```python
from build123d import *

# Parameters (mm, degrees)
SKETCH1_W           = 55.5
SKETCH1_H           = 25
BOSS_EXTRUDE1_DEPTH = 70
SKETCH2_W           = 43.5
SKETCH2_H           = 150
CUT_EXTRUDE1_DEPTH  = 20
SKETCH3_R           = 2
CUT_EXTRUDE2_DEPTH  = 78.910605825
FILLET1_R           = 3
CHAMFER1_SIZE       = 6


with BuildPart() as part:
    # Sketch1 → Boss-Extrude1 (new, symmetric)
    with BuildSketch(Plane.XY):
        Rectangle(SKETCH1_W, SKETCH1_H)
    extrude(amount=BOSS_EXTRUDE1_DEPTH, both=True)

    # Sketch2 → Cut-Extrude1 (cut)
    with BuildSketch(Plane(origin=(0, 12.5, 0), x_dir=(1, 0, 0), z_dir=(0, 1, 0))):
        Rectangle(SKETCH2_W, SKETCH2_H)
    extrude(amount=-CUT_EXTRUDE1_DEPTH, mode=Mode.SUBTRACT)

    # Sketch3 → Cut-Extrude2 (cut, through all)
    with BuildSketch(Plane(origin=(0, -7.5, 0), x_dir=(1, 0, 0), z_dir=(0, 1, 0))):
        with Locations(Location((0, 0, 0), (0, 0, 270))):
            Circle(SKETCH3_R)
    extrude(amount=-CUT_EXTRUDE2_DEPTH, mode=Mode.SUBTRACT)

    # Fillet1
    fillet1_edges = [part.edges().sort_by_distance(p)[0] for p in [
        (27.75, -12.5, 0),
        (-27.75, -12.5, 0),
    ]]
    fillet(fillet1_edges, radius=FILLET1_R)

    # Chamfer1
    # the kernel refuses this chamfer: 6 mm, written as the material it takes off along each edge
    with BuildSketch(Plane(origin=(-6.319902072, 12.5, -70), x_dir=(0, -0.9996219169112968, -0.027495876610586778), z_dir=(-1, 0, 0)), Plane(origin=(43.180097928, 12.5, -70), x_dir=(0, -0.9996219169112968, -0.027495876610586778), z_dir=(-1, 0, 0))) as chamfer1_piece_1:
        Polygon((CHAMFER1_SIZE * 0.999621916911, CHAMFER1_SIZE * 0.0274958766106), (-CHAMFER1_SIZE * 0.0274958766106, CHAMFER1_SIZE * 0.999621916911), (0, 0), align=None)
    extrude(amount=36.860195856, mode=Mode.SUBTRACT)
    with BuildSketch(Plane(origin=(-6.319902072, 12.5, 70), x_dir=(0, -0.9996219169112968, 0.027495876610586778), z_dir=(-1, 0, 0)), Plane(origin=(43.180097928, 12.5, 70), x_dir=(0, -0.9996219169112968, 0.027495876610586778), z_dir=(-1, 0, 0))) as chamfer1_piece_2:
        Polygon((CHAMFER1_SIZE * 0.999621916911, -CHAMFER1_SIZE * 0.0274958766106), (-CHAMFER1_SIZE * 0.0274958766106, -CHAMFER1_SIZE * 0.999621916911), (0, 0), align=None)
    extrude(amount=36.860195856, mode=Mode.SUBTRACT)
    with BuildSketch(Plane(origin=(21.75, 12.5, 85.430097928), x_dir=(-0.027495876610586202, -0.9996219169112968, 0), z_dir=(0, 0, -1)), Plane(origin=(-27.75, 12.5, 85.430097928), x_dir=(-0.027495876610586202, -0.9996219169112968, 0), z_dir=(0, 0, -1)), Plane(origin=(27.75, 12.5, -85.430097928), x_dir=(0.027495876610586202, -0.9996219169112968, 0), z_dir=(0, 0, 1))) as chamfer1_piece_3:
        Polygon((CHAMFER1_SIZE * 0.999621916911, -CHAMFER1_SIZE * 0.0274958766106), (-CHAMFER1_SIZE * 0.0274958766106, -CHAMFER1_SIZE * 0.999621916911), (0, 0), align=None)
    extrude(amount=170.860195856, mode=Mode.SUBTRACT)
    with BuildSketch(Plane(origin=(-21.75, 12.5, -85.430097928), x_dir=(-0.9996219169112969, 0.027495876610586497, 0), z_dir=(0, 0, 1))) as chamfer1_piece_4:
        Polygon((CHAMFER1_SIZE * 0.999621916911, CHAMFER1_SIZE * 0.0274958766106), (-CHAMFER1_SIZE * 0.0274958766106, CHAMFER1_SIZE * 0.999621916911), (0, 0), align=None)
    extrude(amount=170.860195856, mode=Mode.SUBTRACT)


solid = part.part
```
CAD build for the part. Positions are in the model's coordinates, mm. A direction names the side the tool comes from. Give positions to 0.01 mm unless a question says otherwise; leave off trailing zeros. Loops run counter-clockwise (first coordinate to the right, second up) from the corner with the lowest first, then second, coordinate; pieces in that order, holes last. Notation, with made-up numbers: (5, -30.5) -> (44, -30.5) arc R20 cw to (44, 6.5) -> close; hole circle Ø8 at (16, 1). An arc over 180 degrees is marked (long way). Use a Markdown table: item, result.
1. Flat gauge pins, fed straight in: pin 1 (13 mm diameter, centred on x = -5, z = -34, fed in from +Y); pin 2 (12 mm diameter, centred on x = -9.5, y = 1.5, fed in from +Z). Where does each tip first touch, or does it go through?
Check result:
| item | result |
|---|---|
| pin 1 | stops at y = -7.5 |
| pin 2 | passes through |
2. Mould opens along X. For faces 3 (the flat face through (23.23, 7.98, 0.98)), 4 (the cylindrical face through (-26.89, -11.6, 0.98)), 5 (the flat face through (24.8, 7.6, -68.9)), 6 (the cylindrical face through (26.85, -11.64, 0.98)) say: pulls with the +X half, pulls with the -X half, needs draft (parallel to the pull), parting line crosses it, or undercut.
Check result:
| item | result |
|---|---|
| face 3 | undercut |
| face 4 | pulls with the -X half |
| face 5 | needs draft |
| face 6 | pulls with the +X half |
3. Which spindle directions (+Z, -Z, +X, -X, +Y, -Y) get a long thin tool onto all of the face, cutting with end or side? Do faces 1 (the flat face through (5, -7.5, -1)), 2 (the flat face through (27.75, -2, 1)). Say none if no direction does.
Check result:
| item | result |
|---|---|
| face 1 | +Z, -Z, +Y |
| face 2 | +Z, -Z, +X, +Y, -Y |
4. Slice it at A-A (z = 0). List the corners of the cut face in (x, y).
Check result:
| item | result |
|---|---|
| outline | (-27.75, -9.5) arc R3 ccw to (-24.75, -12.5) -> (-2, -12.5) -> (-2, -7.5) -> (-21.75, -7.5) -> (-21.75, 6.5) -> (-24.75, 9.5) -> (-27.75, 6.5) -> close; (2, -12.5) -> (24.75, -12.5) arc R3 ccw to (27.75, -9.5) -> (27.75, 6.5) -> (24.75, 9.5) -> (21.75, 6.5) -> (21.75, -7.5) -> (2, -7.5) -> close |
5. Wall check: L1, parallel to X at y = 6.25, z = -59; L2, parallel to X at y = -9.05, z = 0; L3, parallel to Y at x = -2, z = 33. Give the ranges that are in metal, low to high. Write a range as [from, to].
Check result:
| item | result |
|---|---|
| L1 | x = [-27.75, -21.75], [21.75, 27.75] |
| L2 | x = [-27.75, -2], [2, 27.75] |
| L3 | y = [-12.5, -7.5] |
6. Slice it at D-D (z = 61). List the corners of the cut face in (x, y).
Check result:
| item | result |
|---|---|
| outline | (-27.75, -9.5) arc R3 ccw to (-24.75, -12.5) -> (24.75, -12.5) arc R3 ccw to (27.75, -9.5) -> (27.75, 6.5) -> (24.75, 9.5) -> (21.75, 6.5) -> (21.75, -7.5) -> (-21.75, -7.5) -> (-21.75, 6.5) -> (-24.75, 9.5) -> (-27.75, 6.5) -> close |
7. Slice it at C-C (y = 3.75). List the corners of the cut face in (x, z).
Check result:
| item | result |
|---|---|
| outline | (-27.75, -70) -> (-21.75, -70) -> (-21.75, 70) -> (-27.75, 70) -> close; (21.75, -70) -> (27.75, -70) -> (27.75, 70) -> (21.75, 70) -> close |
8. Slice it at B-B (x = 0). List the corners of the cut face in (y, z).
Check result:
| item | result |
|---|---|
| outline | (-12.5, -70) -> (-7.5, -70) -> (-7.5, -2) -> (-12.5, -2) -> close; (-12.5, 2) -> (-7.5, 2) -> (-7.5, 70) -> (-12.5, 70) -> close |
